```python
from build123d import *

# Parameters (mm, degrees)
F0_R     = 20
F0_R_2   = 15
F1_DEPTH = 7
F2_R     = 20
F3_DEPTH = 3
F4_R     = 4.99999


# Not quite as in the source:
# - a fillet or chamfer is up to 0.001 mm smaller than in the source, because OpenCascade refuses the exact size


with BuildPart() as f1:
    # F0 (on Top) → F1 (new body)
    with BuildSketch(Plane.XY):
        Circle(F0_R)
        Circle(F0_R_2, mode=Mode.SUBTRACT)
    extrude(amount=F1_DEPTH)

    # F2 (on Top) → F3 (join)
    with BuildSketch(Plane.XY):
        Circle(F2_R)
    extrude(amount=-F3_DEPTH)

    # F4 (radius 5 in the source; OpenCascade refuses exactly that, so slightly less here)
    f4_edges = [f1.edges().sort_by_distance(p)[0] for p in [
        (-20, 0, 7),
    ]]
    fillet(f4_edges, radius=F4_R)


solid = f1.part
```
For this review, take the finished solid that the model builds, in its own axes (mm). Give positions to 0.01 mm unless a question says otherwise; leave off trailing zeros. Order: outer loops, then holes, each group sorted by start corner. A loop starts at its lowest first (then second) coordinate and runs counter-clockwise, first axis right, second up.
1) Take a section at B-B (z = 6). Give the boundary of the cut face in (x, y).
2) Insertion check: pin 1 (6 mm diameter, centred on y = -12, z = 1.5, fed in from -X); pin 2 (1 mm diameter, centred on x = 10, y = -8.5, fed in from +Z); pin 3 (1 mm diameter, centred on y = 3, z = -1.5, fed in from +X). Each pin has a flat end and moves straight along its axis. Give the tip position at first contact, or say it passes through.
3) Take a section at D-D (z = -1). Give the boundary of the cut face in (x, y).
4) The part is to be moulded in two halves that separate along X. For faces 1 (the face through (-4.336, -19.524, -0.465)), 2 (the face through (0, 0, -3)), 3 (the face through (-14.985, 0.66, 3.451)), say which applies: released by +X, released by -X, zero draft, split by the parting line, or undercut.
5) Wall thickness on line 1 (Y direction, x = 0, z = 2); line 2 (Z direction, x = -9, y = -4.5); line 3 (Y direction, x = 0, z = 3): over which ranges is each line inside the solid? List them lowest first.
Derived:
1. outline: circle Ø36 at (0, 0); hole circle Ø30 at (0, 0)
2. pin 1: stops at x = -17.86
2. pin 2: stops at z = 0
2. pin 3: stops at x = 19.84
3. outline: circle Ø40 at (0, 0)
4. face 1: split by the parting line
4. face 2: zero draft
4. face 3: undercut
5. line 1: y = -20 to -15, 15 to 20
5. line 2: z = -3 to 0
5. line 3: y = -19.9 to -15, 15 to 19.9
